Check sheet for the modelled part. Datum: model origin and axes. Units: mm. Round coordinates to 2 decimals unless told otherwise and drop trailing zeros. Order: outer loops, then holes, each group sorted by start corner. A loop starts at its lowest first (then second) coordinate and runs counter-clockwise, first axis right, second up. Notation, with made-up numbers: (54, -40) -> (70, -40) arc R17 ccw to (70, -16) -> close; hole circle Ø2 at (61, 44.25). An arc over 180 degrees is marked (long way). Use CSV: the item, a comma, the result in double quotes.
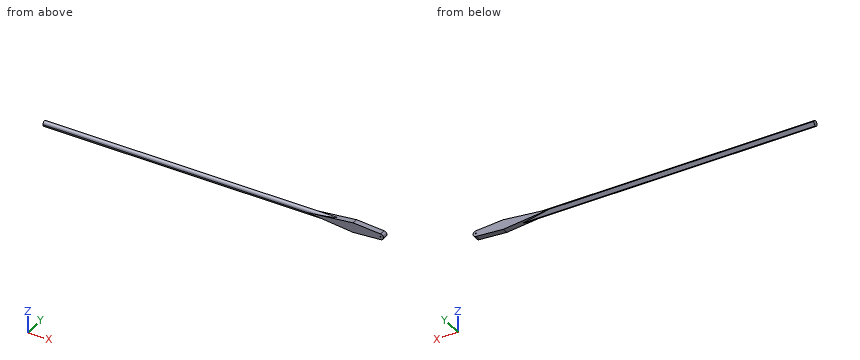
```python
from build123d import *

# Parameters (mm, degrees)
SKETCH1_R           = 1.5
BOSS_EXTRUDE1_DEPTH = 10
CHAMFER1_SIZE       = 10
FILLET1_R           = 10


with BuildPart() as part:
    # Sketch1 → Boss-Extrude1 (new, symmetric)
    with BuildSketch(Plane(origin=(0, 0, 0), x_dir=(1, 0, 0), z_dir=(0, 1, 0))):
        with BuildLine():
            Line((500, 10.00169637), (561.410175266, 16.553276436))
            Line((561.410175266, 16.553276436), (655.434048607, 10.00169637))
            ThreePointArc((655.434048607, 10.00169637), (665.435744977, 0), (655.434048607, -10.00169637))
            Line((655.434048607, -10.00169637), (561.410175266, -16.553276436))
            Line((561.410175266, -16.553276436), (500, -10.00169637))
            Line((500, -10.00169637), (-500, -10.00169637))
            Line((-500, -10.00169637), (-500, 10.00169637))
            Line((-500, 10.00169637), (500, 10.00169637))
        make_face()
        with Locations(Location((655.434048607, 0, 0), (0, 0, 270))):
            Circle(SKETCH1_R, mode=Mode.SUBTRACT)
    extrude(amount=BOSS_EXTRUDE1_DEPTH, both=True)

    # Chamfer1
    chamfer1_edges = [part.edges().sort_by_distance(p)[0] for p in [
        (0, 10, -10.00169637),
        (0, 10, 10.00169637),
    ]]
    chamfer(chamfer1_edges, length=CHAMFER1_SIZE)

    # Fillet1
    fillet1_edges = [part.edges().sort_by_distance(p)[0] for p in [
        (0, -10, 10.00169637),
        (0, -10, -10.00169637),
    ]]
    fillet(fillet1_edges, radius=FILLET1_R - 0.0001)  # a hair under: the kernel refuses the full size


solid = part.part
```
Q1. Scan lines: L1, parallel to X at y = -1, z = 0; L2, parallel to X at y = 2.5, z = -0.5; L3, parallel to Z at x = 328, y = -1. Record each from-to range of solid material in increasing order.
Result sheet:
L1,"x = -500 to 653.93, 656.93 to 665.44"
L2,"x = -500 to 654.02, 656.85 to 665.42"
L3,"z = -9.95 to 9.95"
Q2. Go/stop test with flat-tipped pins: pin 1 (4 mm diameter, centred on x = -270.5, y = 7.5, fed in from +Z); pin 2 (8 mm diameter, centred on x = -54, z = -2, fed in from +Y); pin 3 (8 mm diameter, centred on x = 33.5, y = -2, fed in from -Z); pin 4 (1.8 mm diameter, centred on x = 655.43, z = 0, fed in from +Y). Record where each tip stops, or that it passes through.
Result sheet:
pin 1,"stops at z = 4.5"
pin 2,"stops at y = 10"
pin 3,"stops at z = -10"
pin 4,"passes through"
Q3. Sectioned sample at A-A, the plane y = 3.25. Enter the section's corners in (x, z).
Result sheet:
outline,"(-500, -6.75) -> (469.54, -6.75) -> (561.41, -16.55) -> (655.43, -10) arc R10 ccw to (655.43, 10) -> (561.41, 16.55) -> (469.54, 6.75) -> (-500, 6.75) -> close; hole circle Ø3 at (655.43, 0)"
